```python
from build123d import *

# Parameters (mm, degrees)
SKETCH1_R           = 6
BOSS_EXTRUDE1_DEPTH = 15
SKETCH2_R           = 0.7
CUT_EXTRUDE1_DEPTH  = 3
CIRPATTERN1_COUNT   = 6
FILLET1_R           = 1


with BuildPart() as part:
    # Sketch1 → Boss-Extrude1 (new body)
    with BuildSketch(Plane.XY):
        Circle(SKETCH1_R)
    extrude(amount=BOSS_EXTRUDE1_DEPTH)

    # Sketch2 → Cut-Extrude1 (cut)
    with BuildSketch(Plane.XY.offset(15)):
        with Locations((0, 4.25)):
            Circle(SKETCH2_R)
    cut_extrude1 = extrude(amount=-CUT_EXTRUDE1_DEPTH, mode=Mode.SUBTRACT)

    # CirPattern1: Cut-Extrude1 ×6 about axis
    cirpattern1_axis = Axis((0, 0, 0), (0, 0, 1))
    for i in range(1, CIRPATTERN1_COUNT):
        add(cut_extrude1.rotate(cirpattern1_axis, i * 360 / CIRPATTERN1_COUNT), mode=Mode.SUBTRACT)

    # Fillet1
    fillet1_edges = [part.edges().sort_by_distance(p)[0] for p in [
        (-6, 0, 15),
    ]]
    fillet(fillet1_edges, radius=FILLET1_R)


solid = part.part
```
CAD build for the part. Positions are in the model's coordinates, mm. A direction names the side the tool comes from. Round coordinates to 2 decimals unless told otherwise and drop trailing zeros. Write each loop counter-clockwise with the first axis right and the second up, starting at its lowest first coordinate (ties: lowest second). Pieces come first, ordered by that corner, then holes. Notation, with made-up numbers: (-18, 6.25) -> (13, 6.25) arc R19 ccw to (13, 32.25) -> close; hole circle Ø7 at (24.25, 1). An arc over 180 degrees is marked (long way). Answer in a Markdown table with one row per item. Add a question column.
Item 1: Saw through at A-A, the plane x = 0. Write the cut outline in (y, z), then the cut area to 3 significant figures.
Item 2: Which spindle directions (+Z, -Z, +X, -X, +Y, -Y) get a long thin tool onto all of the face, cutting with end or side? Do faces 1 (the face through (0, 0, 0)), 2 (the face through (-4, 2, 12)). Say none if no direction does.
Item 3: Saw through at B-B, the plane z = 8.5. Write the cut outline in (x, y), then the cut area to 3 significant figures.
Item 4: Mould opens along X. For faces 3 (the face through (0, 0, 15)), 4 (the face through (-6, 0, 7)), 5 (the face through (3.165, -1.652, 13.521)) say: pulls with the +X half, pulls with the -X half, needs draft (parallel to the pull), parting line crosses it, or undercut.
Item 5: Drill centre lines: line 1 (Y direction, x = 0, z = 13.8); line 2 (Y direction, x = 3.5, z = 14); line 3 (Z direction, x = 4.25, y = -2.25). Where is each one in solid material? Low to high. Write a range as from..to.
Item 6: Drop flat-ended pins along their axis: pin 1 Ø2 at (x, y) = (0, 1.5) entering from -Z; pin 2 Ø0.7 at (x, y) = (-3.5, -2) entering from +Z; pin 3 Ø5 at (y, z) = (4.5, 2.5) entering from +X; pin 4 Ø1 at (y, z) = (1, 11.5) entering from -X. Give the stop position or say it passes through.
Findings below:
| question | item | result |
|---|---|---|
| 1 | outline | (-6, 0) -> (6, 0) -> (6, 14) arc R1 ccw to (5, 15) -> (4.95, 15) -> (4.95, 12) -> (3.55, 12) -> (3.55, 15) -> (-3.55, 15) -> (-3.55, 12) -> (-4.95, 12) -> (-4.95, 15) -> (-5, 15) arc R1 ccw to (-6, 14) -> close |
| 1 | area | 171 mm^2 |
| 2 | face 1 | -Z, +X, -X, +Y, -Y |
| 2 | face 2 | +Z |
| 3 | outline | circle Ø12 at (0, 0) |
| 3 | area | 113 mm^2 |
| 4 | face 3 | needs draft |
| 4 | face 4 | parting line crosses it |
| 4 | face 5 | undercut |
| 5 | line 1 | y = -6..-4.95, -3.55..3.55, 4.95..6 |
| 5 | line 2 | y = -4.87..-2.8, -1.45..1.45, 2.8..4.87 |
| 5 | line 3 | z = 0..12 |
| 6 | pin 1 | stops at z = 0 |
| 6 | pin 2 | stops at z = 12 |
| 6 | pin 3 | stops at x = 5.66 |
| 6 | pin 4 | stops at x = -5.98 |
